```python
from build123d import *

# Parameters (mm, degrees)
SKETCH2_R                 = 49.983
MAIN_PART_DEPTH           = 30
MAIN_PART_TAPER           = 1.5
MAIN_PART_OTHER_WAY_DEPTH = 120
MAIN_PART_OTHER_WAY_TAPER = -1.5
SKETCH3_R                 = 47.197422353
MAINCUT_DEPTH             = 150
MAINCUT_DRAFT             = 1.5
FILLET1_R                 = 2


with BuildPart() as part:
    # Sketch2 → Main part (new body)
    with BuildSketch(Plane.XY):
        with Locations((-10.948, 38.989)):
            Circle(SKETCH2_R)
    extrude(amount=MAIN_PART_DEPTH, taper=MAIN_PART_TAPER)

    # Sketch2 → Main part other way (add)
    with BuildSketch(Plane.XY):
        with Locations((-10.948, 38.989)):
            Circle(SKETCH2_R)
    extrude(amount=-MAIN_PART_OTHER_WAY_DEPTH, taper=MAIN_PART_OTHER_WAY_TAPER)


with BuildPart() as maincut_tool:
    # Sketch3 → MainCut (with draft: the straight prism first)
    with BuildSketch(Plane.XY.offset(30)):
        with Locations((-10.948, 38.989)):
            Circle(SKETCH3_R)
    extrude(amount=-MAINCUT_DEPTH)
    # MainCut: the draft: its side faces are tilted about the plane it starts from
    maincut_sides = [maincut_tool.faces().sort_by_distance(p)[0] for p in [
        (-58.145422353, 38.989, -45),
    ]]
    draft(maincut_sides, Plane.XY.offset(30), MAINCUT_DRAFT)


with BuildPart() as part_1:
    add(part.part)

    # MainCut: cut by maincut_tool
    add(maincut_tool.part, mode=Mode.SUBTRACT)

    # Fillet1
    # the kernel refuses this fillet: 2 mm, written as the material it takes off along each edge
    with BuildSketch(Plane(origin=(-10.948, 38.989, -120), x_dir=(1, 0, 0), z_dir=(0, -1, 0))) as fillet1_piece_1:
        with BuildLine():
            CenterArc((53.125310588 - FILLET1_R * 1.02652871406, FILLET1_R), FILLET1_R, 270, 91.5)
            Line((53.125310588 - FILLET1_R * 1.02652871406, 0), (53.125310588, 0))
            Line((53.125310588, 0), (53.125310588 - FILLET1_R * 0.0268713890845, FILLET1_R * 1.02617694831))
        make_face()
    revolve(axis=Axis((-10.948, 38.989, -120), (0, 0, 1)), mode=Mode.SUBTRACT)


solid = part_1.part
```
Part model, mm, in its own coordinate system. Give positions to 0.01 mm unless a question says otherwise; leave off trailing zeros. Order: outer loops, then holes, each group sorted by start corner. A loop starts at its lowest first (then second) coordinate and runs counter-clockwise, first axis right, second up. Notation, with made-up numbers: M 28.25,18.5 L 78.25,18.5 A30 cw 78.25,56.5 Z; hole C 65,15.5 d1. An arc over 180 degrees is marked long. Use a Markdown table: item, result. Add a question column.
(1) Saw through at A-A, the plane z = -91. Give the cut face in (x, y), and give its area (3 significant figures).
(2) Drop flat-ended pins along their axis: P1, Ø1, axis at y = 17.5, z = -33, coming from the +X side; P2, Ø1.5, axis at y = 76, z = -13, coming from the -X side; P3, Ø5, axis at y = 15, z = -16.5, coming from the +X side. Give the stop position or say it passes through.
(3) Probe line 1 along X through (y, z) = (36, -56.5); line 2 along X through (y, z) = (55.5, -63.5); line 3 along Y through (x, z) = (23, 1.5). List the from-to ranges inside material, lowest first. Write a range as [from, to].
(4) Saw through at B-B, the plane z = -69.5. Give the cut face in (x, y).
Answer key:
| question | item | result |
|---|---|---|
| 1 | outline | C -10.95,38.99 d104.73; hole C -10.95,38.99 d100.73 |
| 1 | area | 645 mm^2 |
| 2 | P1 | x = 35.37 |
| 2 | P2 | x = -45.84 |
| 2 | P3 | x = 34.66 |
| 3 | line 1 | [-62.32, -60.32], [38.42, 40.43] |
| 3 | line 2 | [-59.88, -57.77], [35.87, 37.99] |
| 3 | line 3 | [2.36, 5.13], [72.84, 75.62] |
| 4 | outline | C -10.95,38.99 d103.61; hole C -10.95,38.99 d99.61 |
